Geometry check sheet. Reference: drawing and pictorial views, mm from the part's lowest x, y, z. Coordinates: 2 decimals unless noted, no trailing zeros. Loops run counter-clockwise (first coordinate to the right, second up) from the corner with the lowest first, then second, coordinate; pieces in that order, holes last.
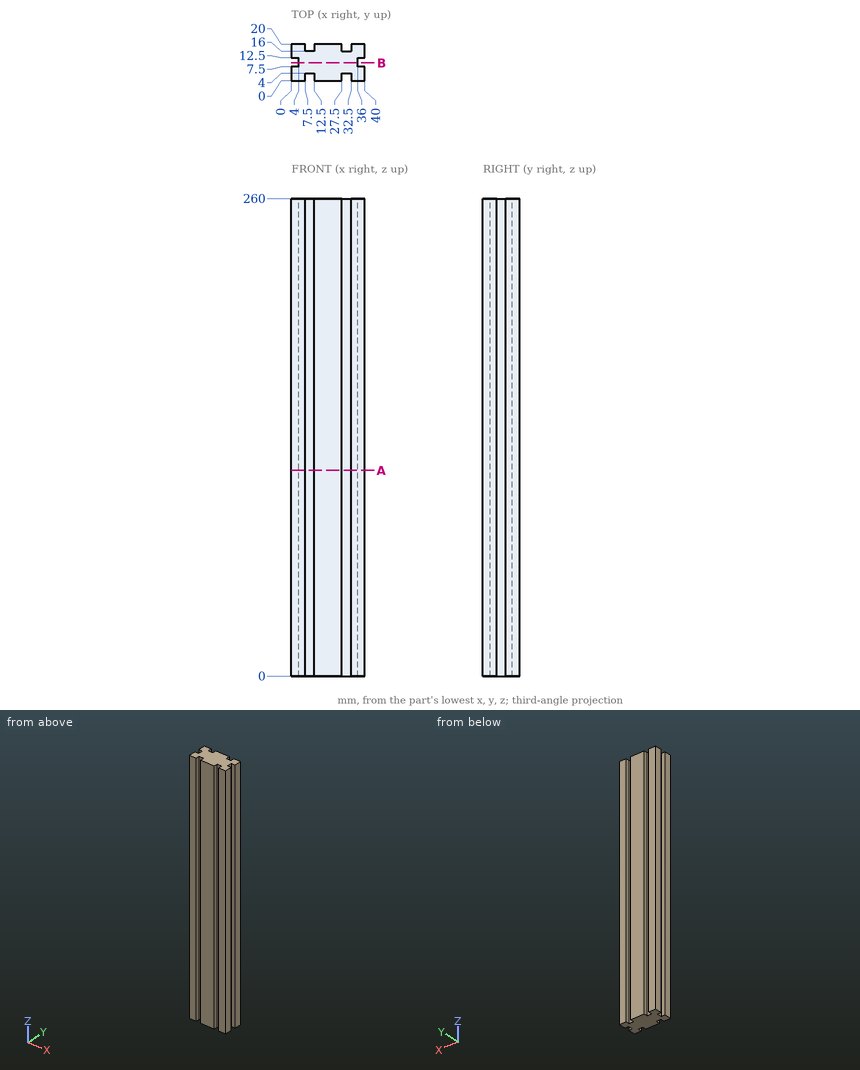
1) Material ranges on probe 1 along X at (y, z) = (2.75, 217.5); probe 2 along Y at (x, z) = (2.5, 110); probe 3 along X at (y, z) = (9.25, 78.5), recorded low to high.
Data:
probe 1: x = 0 to 7.5, 12.5 to 27.5, 32.5 to 40
probe 2: y = 0 to 7.5, 12.5 to 20
probe 3: x = 4 to 36
2) Section check B-B on y = 9.75. Record the cut outline in (x, z), and give its area (3 significant figures).
Data:
outline: (4, 0) - (36, 0) - (36, 260) - (4, 260) - close
area: 8,320 mm2
3) Section check A-A on z = 112. Record the cut outline in (x, y), and give its area (3 significant figures).
Data:
outline: (0, 0) - (7.5, 0) - (7.5, 4) - (12.5, 4) - (12.5, 0) - (27.5, 0) - (27.5, 4) - (32.5, 4) - (32.5, 0) - (40, 0) - (40, 7.5) - (36, 7.5) - (36, 12.5) - (40, 12.5) - (40, 20) - (32.5, 20) - (32.5, 16) - (27.5, 16) - (27.5, 20) - (12.5, 20) - (12.5, 16) - (7.5, 16) - (7.5, 20) - (0, 20) - (0, 12.5) - (4, 12.5) - (4, 7.5) - (0, 7.5) - close
area: 680 mm2
4) Depth check by flat-ended pin: pin 1 (10 mm diameter, centred on x = 30.5, z = 200, fed in from -Y); pin 2 (2.5 mm diameter, centred on x = 31, z = 119, fed in from -Y); pin 3 (3 mm diameter, centred on y = 10.5, z = 162, fed in from +X); pin 4 (2.5 mm diameter, centred on y = 9, z = 154.5, fed in from -X). Enter the tip coordinate at first touch or a pass-through.
Data:
pin 1: stops at y = 0
pin 2: stops at y = 4
pin 3: stops at x = 36
pin 4: stops at x = 4
